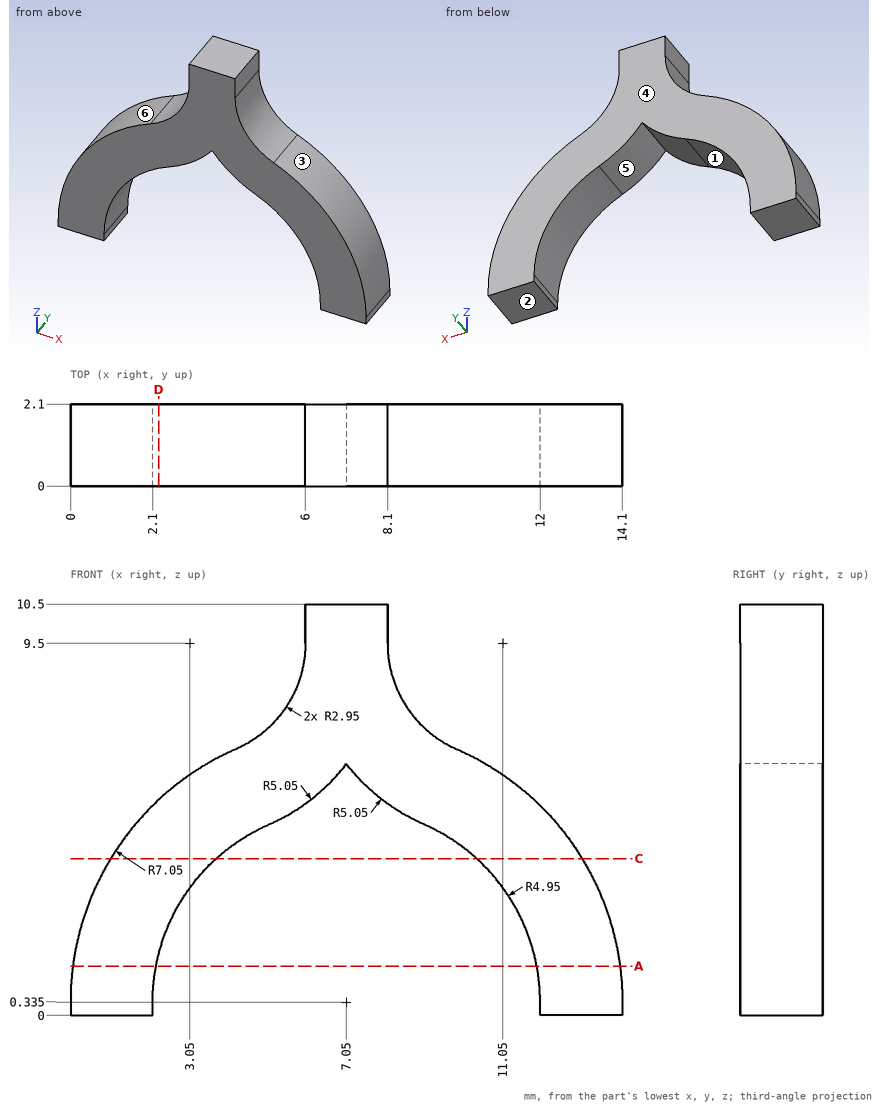
For this review, use the dimensioned drawing (mm, ordinates from the lowest corner) and the shaded views. A direction names the side the tool comes from. Give positions to 0.01 mm unless a question says otherwise; leave off trailing zeros. Write each loop counter-clockwise with the first axis right and the second up, starting at its lowest first coordinate (ties: lowest second). Pieces come first, ordered by that corner, then holes.
(1) For P1, Ø0.5, axis at y = 1.5, z = 10, coming from the -X side; P2, Ø1, axis at x = 3.5, y = 0.5, coming from the +Z side, all flat-tipped, find the tip position at first contact; note any pin that passes through.
(2) Consider section C-C, the plane z = 4. Give the boundary of the cut face in (x, y), and give its area (3 significant figures).
(3) To check wall thickness, follow L1, parallel to X at y = 0.2, z = 5.25 (1 decimal); L2, parallel to X at y = 0.8, z = 1.25 (1 decimal); L3, parallel to X at y = 1.4, z = 9.75. State the ranges of each line that lie inside material, in increasing order.
(4) Consider section A-A, the plane z = 1.25. Give the boundary of the cut face in (x, y).
(5) Consider section D-D, the plane x = 2.25. Give the boundary of the cut face in (y, z).
(6) The part is to be moulded in two halves that separate along X. For the marked faces 3, 4, 5 and 6, say which applies: released by +X, released by -X, zero draft, split by the parting line, or undercut.
(7) Tool access review of the marked faces 1 and 2: name each direction out of +Z, -Z, +X, -X, +Y, -Y from which nothing blocks a thin tool from reaching the whole face with its end or side.
Returned:
1. P1: stops at x = 6
1. P2: stops at z = 6.69
2. outline: (1.03, 0) - (3.72, 0) - (3.72, 2.1) - (1.03, 2.1) - close; (10.38, 0) - (13.07, 0) - (13.07, 2.1) - (10.38, 2.1) - close
2. area: 11.3 mm2
3. L1: x = 2 to 5.8, 8.3 to 12.1
3. L2: x = 0.1 to 2.2, 11.9 to 14
3. L3: x = 6 to 8.1
4. outline: (0.06, 0) - (2.19, 0) - (2.19, 2.1) - (0.06, 2.1) - close; (11.91, 0) - (14.04, 0) - (14.04, 2.1) - (11.91, 2.1) - close
5. outline: (0, 1.54) - (2.1, 1.54) - (2.1, 5.5) - (0, 5.5) - close
6. face 3: released by +X
6. face 4: zero draft
6. face 5: undercut
6. face 6: released by -X
7. face 1: -Z, +Y, -Y
7. face 2: -Z, +X, -X, +Y, -Y
